Answer from the drawing. Dimensions are ordinates in mm from the lowest x, y and z of the part. Round coordinates to 2 decimals unless told otherwise and drop trailing zeros. Loops run counter-clockwise (first coordinate to the right, second up) from the corner with the lowest first, then second, coordinate; pieces in that order, holes last. Notation, with made-up numbers: M 48,-14.75 L 83,-14.75 A18 ccw 83,20.25 Z; hole C 23.5,-11.5 d5. An arc over 180 degrees is marked long. Answer as a JSON object with one key per item and string values.
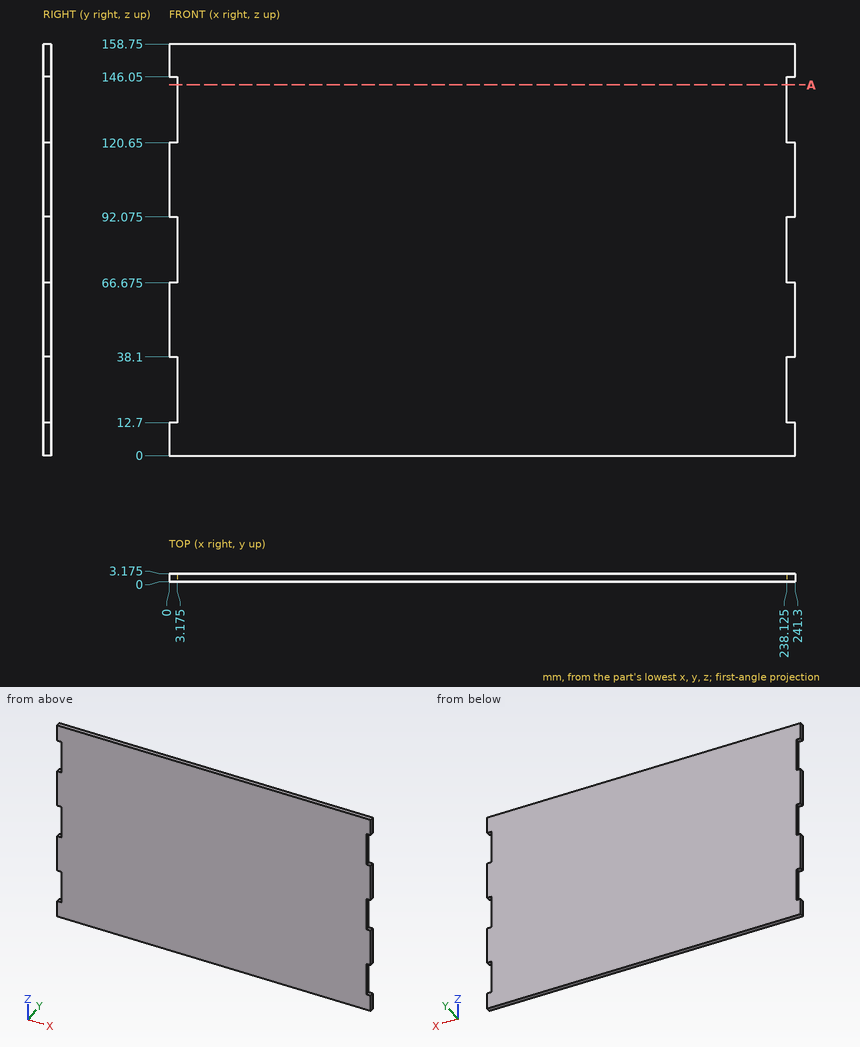
Item 1: Flat-ended cylindrical pins translate along their axes: P1, Ø1.6, axis at y = 1, z = 77, coming from the +X side (3 decimals); P2, Ø1, axis at y = 2, z = 130, coming from the -X side (3 decimals). Find the tip coordinate at first contact, or state that the pin passes through.
Values follow:
{"P1": "x = 238.125", "P2": "x = 3.175"}
Item 2: A straight line is drawn through the part: line 1 (X direction, y = 1.3, z = 73) (3 decimals). Find the intervals that lie inside material, in ascending order.
Values follow:
{"line 1": "3.175 to 238.125"}
Item 3: The part is cut by section A-A (z = 143). Give the vertices of the cut face in (x, y) (3 decimals), then the cut area to 3 significant figures.
Values follow:
{"outline": "M 3.175,0 L 238.125,0 L 238.125,3.175 L 3.175,3.175 Z", "area": "746 mm^2"}
